```python
from build123d import *

# Parameters (mm, degrees)
SKETCH1_R           = 5.078298903
BOSS_EXTRUDE1_DEPTH = 3.175
SKETCH2_R           = 6.35
BOSS_EXTRUDE2_DEPTH = 53.975


with BuildPart() as part:
    # Sketch1 → Boss-Extrude1 (new body)
    with BuildSketch(Plane(origin=(0, 0, 0), x_dir=(1, 0, 0), z_dir=(0, 1, 0))):
        Polygon((-46.777175674, -53.719844845), (-128.460753109, 73.100956593), (-105.319843222, 83.572742001), (-23.636265787, -43.248059437), align=None)
        with Locations((-109.811555345, 67.600325735)):
            Circle(SKETCH1_R, mode=Mode.SUBTRACT)
    extrude(amount=BOSS_EXTRUDE1_DEPTH)

    # Sketch2 → Boss-Extrude2 (add)
    with BuildSketch(Plane(origin=(0, 3.175, 0), x_dir=(1, 0, 0), z_dir=(0, 1, 0))):
        with Locations((-42.032274904, -37.632854988)):
            Circle(SKETCH2_R)
    extrude(amount=-BOSS_EXTRUDE2_DEPTH)


solid = part.part
```
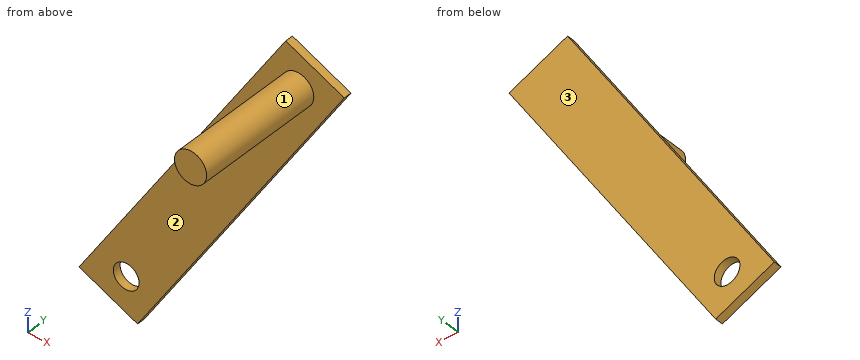
Input: part model. Units: mm. Frame: model coordinates. Face numbers are marked on the shaded views. Give positions to 0.01 mm unless a question says otherwise; leave off trailing zeros. Order: outer loops, then holes, each group sorted by start corner. A loop starts at its lowest first (then second) coordinate and runs counter-clockwise, first axis right, second up. Notation, with made-up numbers: M 7.5,-35.75 L 27.5,-35.75 A10 ccw 27.5,-22.75 Z; hole C 2.5,65.25 d7. An arc over 180 degrees is marked long. One line per question, with ' | ' between items.
1) Section C-C on y = -39. Output: boundary loops of the cut face in (x, z), and give its area (3 significant figures).
Filled in:
outline: C -42.03,37.63 d12.7 | area: 127 mm2
2) Section A-A on x = -41.5. Output: boundary loops of the cut face in (y, z) (1 decimal).
Filled in:
outline: M -50.8,31.3 L 0,31.3 L 0,15.5 L 3.2,15.5 L 3.2,51.3 L 0,51.3 L 0,44 L -50.8,44 Z
3) Section B-B on z = 19.5. Output: boundary loops of the cut face in (x, y) (3 decimals), and give its area (3 significant figures).
Filled in:
outline: M -68.818,0 L -38.932,0 L -38.932,3.175 L -68.818,3.175 Z | area: 94.9 mm2
4) Section D-D on x = -79. Output: boundary loops of the cut face in (y, z) (3 decimals).
Filled in:
outline: M 0,-42.709 L 3.175,-42.709 L 3.175,3.691 L 0,3.691 Z
5) Ray query, L1, parallel to Y at x = -84, z = -40.5 (3 decimals); L2, parallel to Z at x = -45.5, y = -6.5; L3, parallel to X at y = -47, z = 36. Return the intervals inside material, ascending.
Filled in:
L1: y = 0 to 3.175 | L2: z = 32.31 to 42.95 | L3: x = -48.17 to -35.9
6) Contact query for flat-ended pins moving along their axis: P1, Ø11.5, axis at x = -109.81, z = -67.6, coming from the -Y side; P2, Ø3, axis at y = -17, z = 35.5, coming from the -X side. Output: stop coordinate, or through.
Filled in:
P1: stops at y = 0 | P2: stops at x = -48.35
7) Draft query along Y for the marked faces 1, 2 and 3. Return one class per face: pulls with the +Y half, pulls with the -Y half, needs draft (parallel to the pull), parting line crosses it, or undercut.
Filled in:
face 1: needs draft | face 2: pulls with the -Y half | face 3: pulls with the +Y half
